```python
from build123d import *

# Parameters (mm, degrees)
SKETCH_1_R          = 2.1
SKETCH_1_R_2        = 1.6
EXTRUDE_1_DEPTH     = 3
SKETCH_4_W          = 100
SKETCH_4_H          = 3
EXTRUDE_2_DEPTH     = 5
FILLET_1_R          = 5
HOLE_WIZARD_1_D     = 3.5
HOLE_WIZARD_1_DEPTH = 100
SKETCH_5_W          = 12
SKETCH_5_H          = 30
CUT_EXTRUDE_1_DEPTH = 10
HOLE_WIZARD_2_D     = 3


with BuildPart() as part:
    # 草图1 → 凸台-拉伸1 (new body)
    with BuildSketch(Plane(origin=(0, 0, 0), x_dir=(1, 0, 0), z_dir=(0, 1, 0))):
        with BuildLine():
            Line((-31, 0), (31, 0))
            ThreePointArc((31, 0), (45.142135624, 5.857864376), (51, 20))
            Line((51, 20), (51, 60))
            ThreePointArc((51, 60), (51.878679656, 62.121320344), (54, 63))
            Line((54, 63), (92, 63))
            ThreePointArc((92, 63), (94.121320344, 63.878679656), (95, 66))
            Line((95, 66), (95, 136))
            ThreePointArc((95, 136), (94.121320344, 138.121320344), (92, 139))
            Line((92, 139), (-92, 139))
            ThreePointArc((-92, 139), (-94.121320344, 138.121320344), (-95, 136))
            Line((-95, 136), (-95, 66))
            ThreePointArc((-95, 66), (-94.121320344, 63.878679656), (-92, 63))
            Line((-92, 63), (-54, 63))
            ThreePointArc((-54, 63), (-51.878679656, 62.121320344), (-51, 60))
            Line((-51, 60), (-51, 20))
            ThreePointArc((-51, 20), (-45.142135624, 5.857864376), (-31, 0))
        make_face()
        with Locations(Location((-11.75, 23.75, 0), (0, 0, 270))):
            Circle(SKETCH_1_R, mode=Mode.SUBTRACT)
        with Locations(Location((11.75, 23.75, 0), (0, 0, 270))):
            Circle(SKETCH_1_R, mode=Mode.SUBTRACT)
        with Locations(Location((11.75, 6.25, 0), (0, 0, 270))):
            Circle(SKETCH_1_R, mode=Mode.SUBTRACT)
        with Locations(Location((-11.75, 6.25, 0), (0, 0, 270))):
            Circle(SKETCH_1_R, mode=Mode.SUBTRACT)
        with Locations(Location((-61, 71, 0), (0, 0, 270))):
            Circle(SKETCH_1_R_2, mode=Mode.SUBTRACT)
        with Locations(Location((-61, 131, 0), (0, 0, 270))):
            Circle(SKETCH_1_R_2, mode=Mode.SUBTRACT)
        with Locations(Location((-85, 131, 0), (0, 0, 270))):
            Circle(SKETCH_1_R_2, mode=Mode.SUBTRACT)
        with Locations(Location((-85, 71, 0), (0, 0, 270))):
            Circle(SKETCH_1_R_2, mode=Mode.SUBTRACT)
        with Locations(Location((85, 71, 0), (0, 0, 90))):
            Circle(SKETCH_1_R_2, mode=Mode.SUBTRACT)
        with Locations(Location((85, 131, 0), (0, 0, 90))):
            Circle(SKETCH_1_R_2, mode=Mode.SUBTRACT)
        with Locations(Location((61, 131, 0), (0, 0, 90))):
            Circle(SKETCH_1_R_2, mode=Mode.SUBTRACT)
        with Locations(Location((61, 71, 0), (0, 0, 90))):
            Circle(SKETCH_1_R_2, mode=Mode.SUBTRACT)
        with BuildLine():
            Line((-53, 116), (-43, 116))
            ThreePointArc((-43, 116), (-40.878679656, 115.121320344), (-40, 113))
            Line((-40, 113), (-40, 89))
            ThreePointArc((-40, 89), (-40.878679656, 86.878679656), (-43, 86))
            Line((-43, 86), (-53, 86))
            ThreePointArc((-53, 86), (-55.121320344, 86.878679656), (-56, 89))
            Line((-56, 89), (-56, 113))
            ThreePointArc((-56, 113), (-55.121320344, 115.121320344), (-53, 116))
        make_face(mode=Mode.SUBTRACT)
        with BuildLine():
            Line((40, 113), (40, 89))
            ThreePointArc((40, 89), (40.878679656, 86.878679656), (43, 86))
            Line((43, 86), (53, 86))
            ThreePointArc((53, 86), (55.121320344, 86.878679656), (56, 89))
            Line((56, 89), (56, 113))
            ThreePointArc((56, 113), (55.121320344, 115.121320344), (53, 116))
            Line((53, 116), (43, 116))
            ThreePointArc((43, 116), (40.878679656, 115.121320344), (40, 113))
        make_face(mode=Mode.SUBTRACT)
        with BuildLine():
            Line((-20, 89), (20, 89))
            ThreePointArc((20, 89), (23.535533906, 87.535533906), (25, 84))
            Line((25, 84), (25, 44))
            ThreePointArc((25, 44), (23.535533906, 40.464466094), (20, 39))
            Line((20, 39), (-20, 39))
            ThreePointArc((-20, 39), (-23.535533906, 40.464466094), (-25, 44))
            Line((-25, 44), (-25, 84))
            ThreePointArc((-25, 84), (-23.535533906, 87.535533906), (-20, 89))
        make_face(mode=Mode.SUBTRACT)
    extrude(amount=EXTRUDE_1_DEPTH)

    # 草图4 → 凸台-拉伸2 (add)
    with BuildSketch(Plane(origin=(0, 0, -139), x_dir=(-1, 0, 0), z_dir=(0, 0, -1))):
        with Locations((0, 1.5)):
            Rectangle(SKETCH_4_W, SKETCH_4_H)
    extrude(amount=EXTRUDE_2_DEPTH)

    # 圆角1
    fillet_1_edges = [part.edges().sort_by_distance(p)[0] for p in [
        (50, 1.5, -139),
        (-50, 1.5, -139),
    ]]
    fillet(fillet_1_edges, radius=FILLET_1_R - 0.0001)  # a hair under: the kernel refuses the full size

    # 孔1
    with Locations(Plane(origin=(0, 3, 0), x_dir=(1, 0, 0), z_dir=(0, 1, 0))):
        with Locations((-31.8, 134.7), (-31.8, 106.8), (19, 91.6), (20.3, 139.8)):
            Hole(HOLE_WIZARD_1_D / 2, depth=HOLE_WIZARD_1_DEPTH)

    # 草图5 → 切除-拉伸1 (cut)
    with BuildSketch(Plane(origin=(0, 3, 0), x_dir=(1, 0, 0), z_dir=(0, 1, 0))):
        with Locations((-37, 33)):
            Rectangle(SKETCH_5_W, SKETCH_5_H)
    extrude(amount=-CUT_EXTRUDE_1_DEPTH, mode=Mode.SUBTRACT)

    # 孔2 (through all)
    with Locations(Plane(origin=(0, 3, 0), x_dir=(1, 0, 0), z_dir=(0, 1, 0))):
        with Locations((-43, 46.5), (-31, 46.5), (-31, 19.5), (-43, 19.5)):
            Hole(HOLE_WIZARD_2_D / 2)


solid = part.part
```
Work out the finished part from the listing and answer in its coordinate system (mm). A direction names the side the tool comes from. Round coordinates to 2 decimals unless told otherwise and drop trailing zeros. Loops run counter-clockwise (first coordinate to the right, second up) from the corner with the lowest first, then second, coordinate; pieces in that order, holes last. Notation, with made-up numbers: M -17,-15 L 19,-15 A25 ccw 19,12 Z; hole C 38,3.25 d9. An arc over 180 degrees is marked long. One line per question, with ' | ' between items.
Q1. Find section B-B, the plane x = 45. Give the vertices of the cut face in (y, z), then the cut area to 3 significant figures.
Conclusion:
outline: M 0,-144 L 3,-144 L 3,-116 L 0,-116 Z; M 0,-86 L 3,-86 L 3,-5.72 L 0,-5.72 Z | area: 325 mm2
Q2. Find section C-C, the plane y = 0.6. State how many separate pieces and enclosed holes the cut face has, then the cut area to 3 significant figures.
Conclusion:
separate pieces: 1 | enclosed holes: 20 | area: 17,200 mm2
Q3. Each of these flat-tipped pins is pushed along its axis until it touches: pin 1 Ø1.5 at (y, z) = (2, -20) entering from -X; pin 2 Ø0.9 at (y, z) = (1.5, -35) entering from +X; pin 3 Ø1.5 at (x, y) = (75.5, 1) entering from +Z. Where does it stop, or does it pass through?
Conclusion:
pin 1: stops at x = -51 | pin 2: stops at x = 51 | pin 3: stops at z = -63
Q4. Consider line 1 along X through (y, z) = (0.95, -96.5); line 2 along Z through (x, y) = (-85, 1.45); line 3 along X through (y, z) = (0.3, -73). Determine where each line is inside the solid, lowest interval first. Write a range as from..to.
Conclusion:
line 1: x = -95..-56, -40..40, 56..95 | line 2: z = -139..-132.6, -129.4..-72.6, -69.4..-63 | line 3: x = -95..-25, 25..95
Q5. The mould has two halves that part along Z. Classify faces 3 (the flat face through (-1, 0, -105)), 4 (the cylindrical face through (13.832, 1.479, -6.523)), 5 (the cylindrical face through (-52, 2, -140)): +Z half, -Z half, draft (parallel to the pull), parting line (faces both ways), or undercut.
Conclusion:
face 3: draft | face 4: undercut | face 5: -Z half
Q6. Find section A-A, the plane z = -23.75. Give the vertices of the cut face in (x, y), then the cut area to 3 significant figures.
Conclusion:
outline: M -51,0 L -43,0 L -43,3 L -51,3 Z; M -31,0 L -13.85,0 L -13.85,3 L -31,3 Z; M -9.65,0 L 9.65,0 L 9.65,3 L -9.65,3 Z; M 13.85,0 L 51,0 L 51,3 L 13.85,3 Z | area: 245 mm2
Q7. Find section D-D, the plane x = -75. Give the vertices of the cut face in (y, z).
Conclusion:
outline: M 0,-139 L 3,-139 L 3,-63 L 0,-63 Z
Q8. A tool of negligible diameter and unlimited length cuts with its end or side. For faces 1 (the cylindrical face through (52, 2, -140)), 2 (the cylindrical face through (23, 1, -88)), from which of +Z, -Z, +X, -X, +Y, -Y can it reach the whole face along a straight path? Write none if from no direction.
Conclusion:
face 1: -Z, +X, +Y, -Y | face 2: +Y, -Y
